Work out the finished part from the listing and answer in its coordinate system (mm). Face numbers are marked on the shaded views. A direction names the side the tool comes from. Give positions to 0.01 mm unless a question says otherwise; leave off trailing zeros. Write each loop counter-clockwise with the first axis right and the second up, starting at its lowest first coordinate (ties: lowest second). Pieces come first, ordered by that corner, then holes.
1) Find section D-D (y = -0.5). Determine the outline of the cut face in (x, z), plus the area to 3 significant figures.
2) Given pin 1 Ø0.7 at (x, y) = (0, -3.5) entering from +Z; pin 2 Ø0.7 at (y, z) = (-2.5, -2.5) entering from +X; pin 3 Ø0.7 at (x, z) = (-4, 2.5) entering from -Y; pin 4 Ø1 at (x, y) = (-4.5, 1) entering from -Z, each flat-ended and moving along its own axis, determine where each tip first touches the part or whether it passes through.
3) Find section C-C (z = 1.25). Determine the outline of the cut face in (x, y), plus the area to 3 significant figures.
4) Find section B-B (y = -3.25). Determine the outline of the cut face in (x, z), plus the area to 3 significant figures.
5) A tool of negligible diameter and unlimited length cuts with its end or side. For the marked faces 1, 2 and 3, from which of +Z, -Z, +X, -X, +Y, -Y can it reach the whole face along a straight path? Write none if from no direction.
6) Straight lines are drawn through the part: probe 1 along Z at (x, y) = (0, -3); probe 2 along X at (y, z) = (-1, 2.25); probe 3 along Y at (x, z) = (-2, -0.25). For each, find the intervals that lie inside material, in ascending order.
7) Find section A-A (x = -2). Determine the outline of the cut face in (y, z).
```python
from build123d import *

# Parameters (mm, degrees)
SKETCH1_W       = 3
SKETCH1_H       = 2.5
EXTRUDE1_DEPTH  = 4
SKETCH2_W       = 0.645
SKETCH2_H       = 3.5
EXTRUDE2_DEPTH  = 0.64
LPATTERN1_COUNT = 3
LPATTERN1_PITCH = 2.54
CHAMFER1_SIZE   = 0.25


with BuildPart() as part:
    # Sketch1 → Extrude1 (new body, symmetric)
    with BuildSketch(Plane.XY):
        Rectangle(SKETCH1_W, SKETCH1_H)
    extrude(amount=EXTRUDE1_DEPTH, both=True)

    # Sketch2 → Extrude2 (add)
    with BuildSketch(Plane.XY.offset(2.86)):
        with BuildLine():
            Line((-0.3225, 1.25), (-0.3225, 2.245))
            ThreePointArc((-0.3225, 2.245), (-0.374776878, 2.375), (-0.5025, 2.43261663))
            Line((-0.5025, 2.43261663), (-6.5025, 2.43261663))
            Line((-6.5025, 2.43261663), (-6.5025, 3.06831282))
            Line((-6.5025, 3.06831282), (-0.4975, 3.06831282))
            ThreePointArc((-0.4975, 3.06831282), (0.082527742, 2.826), (0.3225, 2.245))
            Line((0.3225, 2.245), (0.3225, 1.25))
            Line((0.3225, 1.25), (-0.3225, 1.25))
        make_face()
        with Locations((0, -3)):
            Rectangle(SKETCH2_W, SKETCH2_H)
    extrude2 = extrude(amount=-EXTRUDE2_DEPTH)

    # LPattern1: Extrude2 ×3
    with Locations(*[(0, 0, -i * LPATTERN1_PITCH) for i in range(1, LPATTERN1_COUNT)]):
        add(extrude2)

    # Chamfer1
    chamfer1_edges = [part.edges().sort_by_distance(p)[0] for p in [
        (-6.5025, 2.750464725, 2.22),
        (-6.5025, 2.43261663, 2.54),
        (-6.5025, 3.06831282, 2.54),
        (-6.5025, 2.750464725, 2.86),
        (0, -4.75, 2.22),
        (0.3225, -4.75, 2.54),
        (-0.3225, -4.75, 2.54),
        (0, -4.75, 2.86),
        (-6.5025, 2.750464725, -0.32),
        (-6.5025, 2.43261663, 0),
        (-6.5025, 3.06831282, 0),
        (-6.5025, 2.750464725, 0.32),
        (0, -4.75, -0.32),
        (0.3225, -4.75, 0),
        (-0.3225, -4.75, 0),
        (0, -4.75, 0.32),
        (-6.5025, 2.750464725, -2.86),
        (-6.5025, 2.43261663, -2.54),
        (-6.5025, 3.06831282, -2.54),
        (-6.5025, 2.750464725, -2.22),
        (0, -4.75, -2.86),
        (0.3225, -4.75, -2.54),
        (-0.3225, -4.75, -2.54),
        (0, -4.75, -2.22),
    ]]
    chamfer(chamfer1_edges, length=CHAMFER1_SIZE)


solid = part.part
```
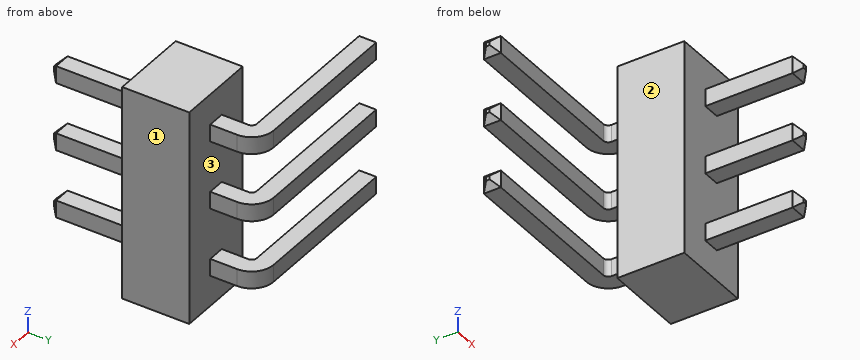
Results:
1. outline: (-1.5, -4) - (1.5, -4) - (1.5, 4) - (-1.5, 4) - close
1. area: 24.0 mm2
2. pin 1: stops at z = 2.86
2. pin 2: stops at x = 0.32
2. pin 3: stops at y = 2.43
2. pin 4: passes through
3. outline: (-1.5, -1.25) - (1.5, -1.25) - (1.5, 1.25) - (-1.5, 1.25) - close
3. area: 7.50 mm2
4. outline: (-0.32, -2.86) - (0.32, -2.86) - (0.32, -2.22) - (-0.32, -2.22) - close; (-0.32, -0.32) - (0.32, -0.32) - (0.32, 0.32) - (-0.32, 0.32) - close; (-0.32, 2.22) - (0.32, 2.22) - (0.32, 2.86) - (-0.32, 2.86) - close
4. area: 1.24 mm2
5. face 1: +Z, -Z, +X, +Y, -Y
5. face 2: +Z, -Z, -X, -Y
5. face 3: none
6. probe 1: z = -2.86 to -2.22, -0.32 to 0.32, 2.22 to 2.86
6. probe 2: x = -1.5 to 1.5
6. probe 3: y = 2.43 to 3.07
7. outline: (2.43, -2.86) - (3.07, -2.86) - (3.07, -2.22) - (2.43, -2.22) - close; (2.43, -0.32) - (3.07, -0.32) - (3.07, 0.32) - (2.43, 0.32) - close; (2.43, 2.22) - (3.07, 2.22) - (3.07, 2.86) - (2.43, 2.86) - close
